```python
from build123d import *

# Parameters (mm, degrees)
SKETCH_W        = 40
SKETCH_H        = 51
PAD_DEPTH       = 7
SKETCH001_W     = 35
SKETCH001_H     = 46
POCKET_DEPTH    = 5
SKETCH002_W     = 44
SKETCH002_H     = 55
PAD001_DEPTH    = 3
SKETCH003_W     = 44
SKETCH003_H     = 55
SKETCH003_W_2   = 40
SKETCH003_H_2   = 51
PAD002_DEPTH    = 50
SKETCH004_R     = 1.3
SKETCH004_W     = 27.5
SKETCH004_H     = 19.2
POCKET001_DEPTH = 5
SKETCH005_R     = 2
POCKET002_DEPTH = 5
SKETCH006_R     = 1.6
SKETCH006_W     = 15.5
SKETCH006_H     = 22
POCKET003_DEPTH = 5


with BuildPart() as part:
    # Sketch → Pad (new body)
    with BuildSketch(Plane.XY):
        with Locations((20, 25.5)):
            Rectangle(SKETCH_W, SKETCH_H)
    extrude(amount=PAD_DEPTH)

    # Sketch001 → Pocket (cut)
    with BuildSketch(Plane.XY.offset(7)):
        with Locations((20, 25.5)):
            Rectangle(SKETCH001_W, SKETCH001_H)
    extrude(amount=-POCKET_DEPTH, mode=Mode.SUBTRACT)

    # Sketch002 → Pad001 (new body)
    with BuildSketch(Plane(origin=(0, 0, 0), x_dir=(1, 0, 0), z_dir=(0, 0, -1))):
        with Locations((20, -25.5)):
            Rectangle(SKETCH002_W, SKETCH002_H)
    extrude(amount=PAD001_DEPTH)

    # Sketch003 → Pad002 (new body)
    with BuildSketch(Plane.XY):
        with Locations((20, 25.5)):
            Rectangle(SKETCH003_W, SKETCH003_H)
        with Locations((20, 25.5)):
            Rectangle(SKETCH003_W_2, SKETCH003_H_2, mode=Mode.SUBTRACT)
    extrude(amount=PAD002_DEPTH)

    # Sketch004 → Pocket001 (cut)
    with BuildSketch(Plane.XZ.offset(2)):
        with Locations((11.591859, 22.0259)):
            Circle(SKETCH004_R)
        with Locations((32.291859, 22.0259)):
            Circle(SKETCH004_R)
        with Locations((11.591859, 45.4259)):
            Circle(SKETCH004_R)
        with Locations((32.291859, 45.4259)):
            Circle(SKETCH004_R)
        with Locations((20, 33.6)):
            Rectangle(SKETCH004_W, SKETCH004_H)
    extrude(amount=-POCKET001_DEPTH, mode=Mode.SUBTRACT)

    # Sketch005 → Pocket002 (cut)
    with BuildSketch(Plane.XZ.offset(2)):
        with Locations((11, 13)):
            Circle(SKETCH005_R)
        with Locations((20, 13)):
            Circle(SKETCH005_R)
        with Locations((29, 13)):
            Circle(SKETCH005_R)
    extrude(amount=-POCKET002_DEPTH, mode=Mode.SUBTRACT)

    # Sketch006 → Pocket003 (cut)
    with BuildSketch(Plane(origin=(-2, 0, 0), x_dir=(0, -1, 0), z_dir=(-1, 0, 0))):
        with Locations((-39.811333, 43.678651)):
            Circle(SKETCH006_R)
        with Locations((-39.817526, 30.238866)):
            Rectangle(SKETCH006_W, SKETCH006_H)
    extrude(amount=-POCKET003_DEPTH, mode=Mode.SUBTRACT)


solid = part.part
```
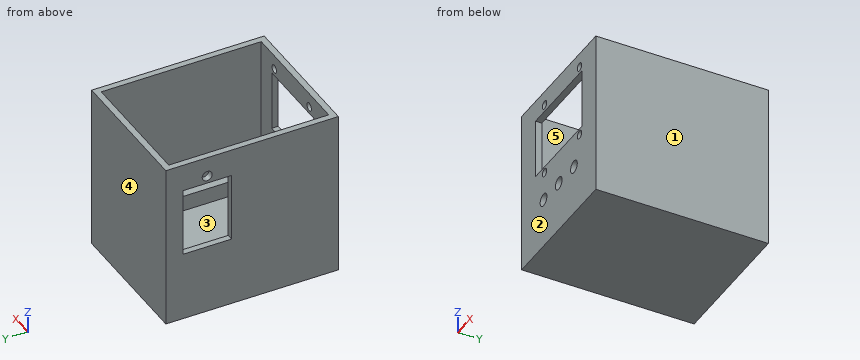
Geometry: final body of the model. Coordinates: model frame, mm. Face numbers are marked on the shaded views. A direction names the side the tool comes from. Round coordinates to 2 decimals unless told otherwise and drop trailing zeros. Loops run counter-clockwise (first coordinate to the right, second up) from the corner with the lowest first, then second, coordinate; pieces in that order, holes last. Notation, with made-up numbers: (24.25, 51.25) -> (67.25, 51.25) arc R22 cw to (67.25, 67.25) -> close; hole circle Ø4 at (69.25, 56). An arc over 180 degrees is marked (long way). Use one line per item in the form item = value. Start each with the question number.
1) Draft query along Y for the marked faces 1, 2 and 3. Return one class per face: released by +Y, released by -Y, zero draft, split by the parting line, or undercut.
2) Access query for the marked faces 4 and 5. Directions: +Z, -Z, +X, -X, +Y, -Y. A direction counts if a zero-diameter tool reaches every point of the face in a straight line with its end or side. Return the directions, or none.
3) Section C-C on z = 13. Output: boundary loops of the cut face in (x, y), then the cut area to 3 significant figures.
4) Section A-A on y = 43. Output: boundary loops of the cut face in (x, z), then the cut area to 3 significant figures.
5) Section B-B on x = 20. Output: boundary loops of the cut face in (y, z), then the cut area to 3 significant figures.
6) Line query: L1, parallel to Z at x = 20, y = -0.85; L2, parallel to Y at x = 21, z = 17; L3, parallel to X at y = 13.5, z = 33.5. Output: solid intervals per line, ascending.
7) First-contact query: P1, Ø6, axis at x = 9, y = 13.5, coming from the +Z side; P2, Ø2, axis at x = 10.5, z = 28, coming from the -Y side. Flat tips, straight axial feed; report the tip coordinate or a pass-through.
8) Section D-D on z = 29.5. Output: boundary loops of the cut face in (x, y).
Response:
q1.face_1 = zero draft
q1.face_2 = released by -Y
q1.face_3 = undercut
q2.face_4 = +Z, -Z, +X, -X, +Y
q2.face_5 = +Z
q3.outline = (-2, -2) -> (9, -2) -> (9, 0) -> (0, 0) -> (0, 51) -> (40, 51) -> (40, 0) -> (31, 0) -> (31, -2) -> (42, -2) -> (42, 53) -> (-2, 53) -> close; (13, -2) -> (18, -2) -> (18, 0) -> (13, 0) -> close; (22, -2) -> (27, -2) -> (27, 0) -> (22, 0) -> close
q3.area = 356 mm^2
q4.outline = (-2, -3) -> (42, -3) -> (42, 50) -> (40, 50) -> (40, 7) -> (37.5, 7) -> (37.5, 2) -> (2.5, 2) -> (2.5, 7) -> (0, 7) -> (0, 19.24) -> (-2, 19.24) -> close; (-2, 41.24) -> (0, 41.24) -> (0, 50) -> (-2, 50) -> close
q4.area = 393 mm^2
q5.outline = (-2, -3) -> (53, -3) -> (53, 50) -> (51, 50) -> (51, 7) -> (48.5, 7) -> (48.5, 2) -> (2.5, 2) -> (2.5, 7) -> (0, 7) -> (0, 11) -> (-2, 11) -> close; (-2, 15) -> (0, 15) -> (0, 24) -> (-2, 24) -> close; (-2, 43.2) -> (0, 43.2) -> (0, 50) -> (-2, 50) -> close
q5.area = 446 mm^2
q6.L1 = -3 to 11, 15 to 24, 43.2 to 50
q6.L2 = -2 to 0, 51 to 53
q6.L3 = -2 to 0, 40 to 42
q7.P1 = 2
q7.P2 = 51
q8.outline = (-2, -2) -> (6.25, -2) -> (6.25, 0) -> (0, 0) -> (0, 32.07) -> (-2, 32.07) -> close; (-2, 47.57) -> (0, 47.57) -> (0, 51) -> (40, 51) -> (40, 0) -> (33.75, 0) -> (33.75, -2) -> (42, -2) -> (42, 53) -> (-2, 53) -> close
